```python
from build123d import *

# Parameters (mm, degrees)
SKETCH1_R           = 1.4
BOSS_EXTRUDE1_DEPTH = 3


with BuildPart() as part:
    # Sketch1 → Boss-Extrude1 (new body)
    with BuildSketch(Plane(origin=(0, 0, 0), x_dir=(1, 0, 0), z_dir=(0, 1, 0))):
        with BuildLine():
            Line((-76.22405565, 13.400206277), (-57.554638622, 12))
            Line((-57.554638622, 12), (-5.000314195, 12))
            ThreePointArc((-5.000314195, 12), (-2.878993852, 11.121320344), (-2.000314195, 9))
            Line((-2.000314195, 9), (-2.000314195, -9.00840207))
            ThreePointArc((-2.000314195, -9.00840207), (-2.878993852, -11.129722414), (-5.000314195, -12.00840207))
            Line((-5.000314195, -12.00840207), (-57.779008466, -12.00840207))
            Line((-57.779008466, -12.00840207), (-76.22468404, -13.391827738))
            ThreePointArc((-76.22468404, -13.391827738), (-78.199531048, -14.342973455), (-79.000314195, -16.383425668))
            Line((-79.000314195, -16.383425668), (-79.000314195, -25))
            ThreePointArc((-79.000314195, -25), (-75.000314195, -29), (-71.000314195, -25))
            Line((-71.000314195, -25), (-71.000314195, -23))
            ThreePointArc((-71.000314195, -23), (-70.121634539, -20.878679656), (-68.000314195, -20))
            Line((-68.000314195, -20), (-7.000314195, -20))
            ThreePointArc((-7.000314195, -20), (-4.878993852, -20.878679656), (-4.000314195, -23))
            Line((-4.000314195, -23), (-4.000314195, -25))
            ThreePointArc((-4.000314195, -25), (-0.000314195, -29), (3.999685805, -25))
            Line((3.999685805, -25), (3.999685805, -23))
            ThreePointArc((3.999685805, -23), (4.878365461, -20.878679656), (6.999685805, -20))
            Line((6.999685805, -20), (67.999057414, -20))
            ThreePointArc((67.999057414, -20), (70.120377758, -20.878679656), (70.999057414, -23))
            Line((70.999057414, -23), (70.999057414, -25))
            ThreePointArc((70.999057414, -25), (74.999057414, -29), (78.999057414, -25))
            Line((78.999057414, -25), (78.999057414, -16.391804207))
            ThreePointArc((78.999057414, -16.391804207), (78.198274268, -14.351351994), (76.223427259, -13.400206277))
            Line((76.223427259, -13.400206277), (57.554010231, -12))
            Line((57.554010231, -12), (20.999685805, -12))
            ThreePointArc((20.999685805, -12), (18.878365461, -11.121320344), (17.999685805, -9))
            Line((17.999685805, -9), (17.999685805, 9.00840207))
            ThreePointArc((17.999685805, 9.00840207), (18.878365461, 11.129722414), (20.999685805, 12.00840207))
            Line((20.999685805, 12.00840207), (57.778380076, 12.00840207))
            Line((57.778380076, 12.00840207), (76.22405565, 13.391827738))
            ThreePointArc((76.22405565, 13.391827738), (78.199300731, 14.342772308), (79.000314195, 16.383425668))
            Line((79.000314195, 16.383425668), (79.000314195, 25))
            ThreePointArc((79.000314195, 25), (75.000314195, 29), (71.000314195, 25))
            Line((71.000314195, 25), (71.000314195, 23))
            ThreePointArc((71.000314195, 23), (70.121634539, 20.878679656), (68.000314195, 20))
            Line((68.000314195, 20), (7.000314195, 20))
            ThreePointArc((7.000314195, 20), (4.878993852, 20.878679656), (4.000314195, 23))
            Line((4.000314195, 23), (4.000314195, 25))
            ThreePointArc((4.000314195, 25), (0.000314195, 29), (-3.999685805, 25))
            Line((-3.999685805, 25), (-3.999685805, 23))
            ThreePointArc((-3.999685805, 23), (-4.878365461, 20.878679656), (-6.999685805, 20))
            Line((-6.999685805, 20), (-67.999685805, 20))
            ThreePointArc((-67.999685805, 20), (-70.121006148, 20.878679656), (-70.999685805, 23))
            Line((-70.999685805, 23), (-70.999685805, 25))
            ThreePointArc((-70.999685805, 25), (-74.999685805, 29), (-78.999685805, 25))
            Line((-78.999685805, 25), (-78.999685805, 16.391804207))
            ThreePointArc((-78.999685805, 16.391804207), (-78.198902658, 14.351351994), (-76.22405565, 13.400206277))
        make_face()
        with Locations((74.999685805, 25)):
            Circle(SKETCH1_R, mode=Mode.SUBTRACT)
        with Locations((74.999685805, -25)):
            Circle(SKETCH1_R, mode=Mode.SUBTRACT)
        with Locations((-0.000314195, -25)):
            Circle(SKETCH1_R, mode=Mode.SUBTRACT)
        with Locations((-0.000314195, 25)):
            Circle(SKETCH1_R, mode=Mode.SUBTRACT)
        with Locations((-75.000314195, 25)):
            Circle(SKETCH1_R, mode=Mode.SUBTRACT)
        with Locations((-75.000314195, -25)):
            Circle(SKETCH1_R, mode=Mode.SUBTRACT)
        with BuildLine():
            Line((55.499685805, -17.5), (50.499685805, -17.5))
            ThreePointArc((50.499685805, -17.5), (48.999685805, -16), (50.499685805, -14.5))
            Line((50.499685805, -14.5), (55.499685805, -14.5))
            ThreePointArc((55.499685805, -14.5), (56.999685805, -16), (55.499685805, -17.5))
        make_face(mode=Mode.SUBTRACT)
        with BuildLine():
            Line((50.499685805, 17.5), (55.499685805, 17.5))
            ThreePointArc((55.499685805, 17.5), (56.999685805, 16), (55.499685805, 14.5))
            Line((55.499685805, 14.5), (50.499685805, 14.5))
            ThreePointArc((50.499685805, 14.5), (48.999685805, 16), (50.499685805, 17.5))
        make_face(mode=Mode.SUBTRACT)
        with BuildLine():
            Line((12.999685805, 2), (12.999685805, -2))
            ThreePointArc((12.999685805, -2), (7.999685805, -7), (2.999685805, -2))
            Line((2.999685805, -2), (2.999685805, 2))
            ThreePointArc((2.999685805, 2), (7.999685805, 7), (12.999685805, 2))
        make_face(mode=Mode.SUBTRACT)
        with BuildLine():
            Line((-49.500314195, -17.5), (-54.500314195, -17.5))
            ThreePointArc((-54.500314195, -17.5), (-56.000314195, -16), (-54.500314195, -14.5))
            Line((-54.500314195, -14.5), (-49.500314195, -14.5))
            ThreePointArc((-49.500314195, -14.5), (-48.000314195, -16), (-49.500314195, -17.5))
        make_face(mode=Mode.SUBTRACT)
        with BuildLine():
            Line((-54.500314195, 17.5), (-49.500314195, 17.5))
            ThreePointArc((-49.500314195, 17.5), (-48.000314195, 16), (-49.500314195, 14.5))
            Line((-49.500314195, 14.5), (-54.500314195, 14.5))
            ThreePointArc((-54.500314195, 14.5), (-56.000314195, 16), (-54.500314195, 17.5))
        make_face(mode=Mode.SUBTRACT)
    extrude(amount=BOSS_EXTRUDE1_DEPTH)


solid = part.part
```
Here's how the part is built. I have some questions about the finished solid (model axes, mm). A direction names the side the tool comes from. Give positions to 0.01 mm unless a question says otherwise; leave off trailing zeros. Loops run counter-clockwise (first coordinate to the right, second up) from the corner with the lowest first, then second, coordinate; pieces in that order, holes last. Notation, with made-up numbers: (86, -12.5) -> (108, -12.5) arc R20 ccw to (108, 14.5) -> close; hole circle Ø1 at (59, 27). An arc over 180 degrees is marked (long way). Use one line per item in the form item = value. Start each with the question number.
1) For P1, Ø0.9, axis at x = 32, y = 1.5, coming from the -Z side; P2, Ø0.9, axis at x = -47.5, y = 1.5, coming from the +Z side, each with a flat end and sliding along its axis, tell me the tip position at first contact or that it passes through.
2) Imagine slicing it at C-C (y = 0.45). Count the separate pieces of the cut face and the enclosed holes in it, then the cut area to 3 significant figures.
3) Thinking about a two-plate mould opening in Z: for faces 4 (the face through (0, 1, 29)), 5 (the face through (13, 1, 0)), 6 (the face through (4.9, 1.48, -20.86)), which applies, +Z half, -Z half, draft (parallel to the pull), parting line (faces both ways), or undercut?
4) Imagine slicing it at B-B (z = -3.5). Please give me the cut outline in (x, y), then the cut area to 3 significant figures.
5) Which directions (+Z, -Z, +X, -X, +Y, -Y) give clear straight access to the entire face, cutting with the end or side of a thin tool? Please do faces 1 (the face through (57, 1, 16)), 2 (the face through (4.86, 1.48, 20.9)), 3 (the face through (39, 1, -12.008)).
6) Imagine slicing it at A-A (x = -17). Please give me the cut outline in (y, z).
7) Please list where these lines run through material, in increasing order: line 1 along Z through (x, y) = (-53.5, 0.55); line 2 along X through (y, z) = (0.8, 25); line 3 along Z through (x, y) = (39, 1.45).
Check values:
q1.P1 = -20
q1.P2 = 20
q2.separate_pieces = 1
q2.enclosed_holes = 11
q2.area = 3,100 mm^2
q3.face_4 = +Z half
q3.face_5 = undercut
q3.face_6 = -Z half
q4.outline = (-2, 0) -> (3.23, 0) -> (3.23, 3) -> (-2, 3) -> close; (12.77, 0) -> (18, 0) -> (18, 3) -> (12.77, 3) -> close
q4.area = 31.4 mm^2
q5.face_1 = +Y, -Y
q5.face_2 = +Z, +Y, -Y
q5.face_3 = +X, +Y, -Y
q6.outline = (0, -20) -> (3, -20) -> (3, -12) -> (0, -12) -> close; (0, 12.01) -> (3, 12.01) -> (3, 20) -> (0, 20) -> close
q7.line_1 = -20 to -17.5, -14.5 to -12, 12.01 to 14.5, 17.5 to 20
q7.line_2 = -79 to -76.4, -73.6 to -71, -4 to -1.4, 1.4 to 4, 71 to 73.6, 76.4 to 79
q7.line_3 = -20 to -12.01, 12 to 20
